Input: part model. Units: mm. Frame: model coordinates. Face numbers are marked on the shaded views. A direction names the side the tool comes from. Give positions to 0.01 mm unless a question says otherwise; leave off trailing zeros. Loops run counter-clockwise (first coordinate to the right, second up) from the corner with the lowest first, then second, coordinate; pieces in that order, holes last. Notation, with made-up numbers: (16.25, -19) - (57.25, -19) arc R13 cw to (57.25, 2) - close; hole circle Ø4 at (-38, 59.25). An arc over 180 degrees is marked (long way). One line per item, written item: value.
from build123d import *

# Parameters (mm, degrees)
ESBO_O1_W                = 37
ESBO_O1_H                = 17
RESSALTO_EXTRUS_O1_DEPTH = 0.45
ESBO_O2_W                = 10
ESBO_O2_H                = 11
RESSALTO_EXTRUS_O2_DEPTH = 5.1
RESSALTO_EXTRUS_O3_DEPTH = 5.1
ESBO_O4_W                = 4
ESBO_O4_H                = 1.5
CORTE_EXTRUS_O1_DEPTH    = 0.1
CHANFRO1_SIZE            = 1


with BuildPart() as part:
    # Esboço1 → Ressalto-extrusão1 (new, symmetric)
    with BuildSketch(Plane(origin=(0, 0, 0), x_dir=(1, 0, 0), z_dir=(0, 1, 0))):
        Rectangle(ESBO_O1_W, ESBO_O1_H)
    extrude(amount=RESSALTO_EXTRUS_O1_DEPTH, both=True)

    # Esboço2 → Ressalto-extrusão2 (add)
    with BuildSketch(Plane(origin=(0, 0.45, 0), x_dir=(1, 0, 0), z_dir=(0, 1, 0))):
        with Locations((-6.5, -2)):
            Rectangle(ESBO_O2_W, ESBO_O2_H)
    extrude(amount=RESSALTO_EXTRUS_O2_DEPTH)

    # Esboço3 → Ressalto-extrusão3 (add)
    with BuildSketch(Plane(origin=(0, 0.45, 0), x_dir=(1, 0, 0), z_dir=(0, 1, 0))):
        Polygon((0.5, 0.910833496), (0.5, 6.089166504), (1.910833496, 7.5), (8.967936907, 7.5), (9.5, 6.967936907), (9.5, 0.62041406), (8.37958594, -0.5), (1.910833496, -0.5), align=None)
    extrude(amount=RESSALTO_EXTRUS_O3_DEPTH)

    # Esboço4 → Corte-extrusão1 (cut)
    with BuildSketch(Plane(origin=(0, 0.45, 0), x_dir=(1, 0, 0), z_dir=(0, 1, 0))):
        with Locations((-15, 4.75)):
            Rectangle(ESBO_O4_W, ESBO_O4_H)
        with Locations((-15, -4.75)):
            Rectangle(ESBO_O4_W, ESBO_O4_H)
        with Locations((15, -4.75)):
            Rectangle(ESBO_O4_W, ESBO_O4_H)
        with Locations((15, 4.75)):
            Rectangle(ESBO_O4_W, ESBO_O4_H)
    extrude(amount=-CORTE_EXTRUS_O1_DEPTH, mode=Mode.SUBTRACT)

    # Chanfro1
    chanfro1_edges = [part.edges().sort_by_distance(p)[0] for p in [
        (-18.5, 0, -8.5),
        (18.5, 0, -8.5),
        (18.5, 0, 8.5),
        (-18.5, 0, 8.5),
    ]]
    chamfer(chanfro1_edges, length=CHANFRO1_SIZE)


solid = part.part
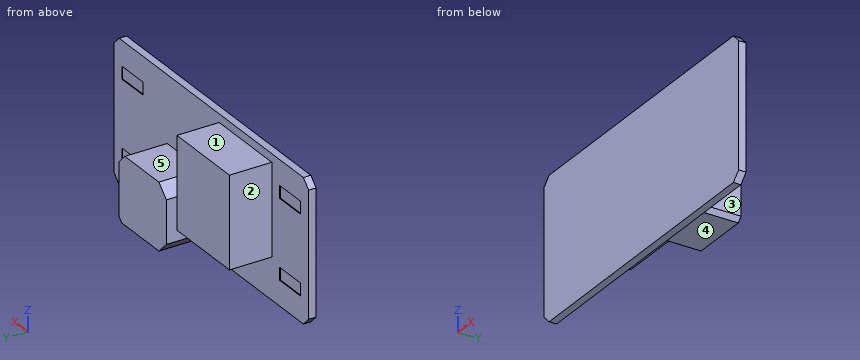
Item 1: Access query for the marked faces 1, 2, 3, 4 and 5. Directions: +Z, -Z, +X, -X, +Y, -Y. A direction counts if a zero-diameter tool reaches every point of the face in a straight line with its end or side. Return the directions, or none.
Verdict:
face 1: +Z, +X, -X, +Y
face 2: +Z, -Z, -X, +Y
face 3: +Z, -Z, +X, +Y
face 4: -Z, +X, -X, +Y
face 5: +Z, +X, +Y
Item 2: Section D-D, the plane z = 3.5. Output: boundary loops of the cut face in (x, y), and give its area (3 significant figures).
Verdict:
outline: (-18.5, -0.45) - (18.5, -0.45) - (18.5, 0.45) - (-1.5, 0.45) - (-1.5, 5.55) - (-11.5, 5.55) - (-11.5, 0.45) - (-18.5, 0.45) - close
area: 84.3 mm^2
Item 3: Section A-A, the plane y = 3.1. Output: boundary loops of the cut face in (x, z), and give its area (3 significant figures).
Verdict:
outline: (-11.5, -3.5) - (-1.5, -3.5) - (-1.5, 7.5) - (-11.5, 7.5) - close; (0.5, -6.09) - (1.91, -7.5) - (8.97, -7.5) - (9.5, -6.97) - (9.5, -0.62) - (8.38, 0.5) - (1.91, 0.5) - (0.5, -0.91) - close
area: 179 mm^2
Item 4: Section C-C, the plane z = -4.5. Output: boundary loops of the cut face in (x, y).
Verdict:
outline: (-18.5, -0.45) - (18.5, -0.45) - (18.5, 0.45) - (17, 0.45) - (17, 0.35) - (13, 0.35) - (13, 0.45) - (9.5, 0.45) - (9.5, 5.55) - (0.5, 5.55) - (0.5, 0.45) - (-13, 0.45) - (-13, 0.35) - (-17, 0.35) - (-17, 0.45) - (-18.5, 0.45) - close
Item 5: Section B-B, the plane x = 4. Output: boundary loops of the cut face in (y, z).
Verdict:
outline: (-0.45, -8.5) - (0.45, -8.5) - (0.45, -7.5) - (5.55, -7.5) - (5.55, 0.5) - (0.45, 0.5) - (0.45, 8.5) - (-0.45, 8.5) - close
Item 6: Pin query (flat end, axial travel): P1, Ø8, axis at x = -12, z = 1.5, coming from the +Y side; P2, Ø2.5, axis at x = -8.5, y = 4, coming from the +Z side; P3, Ø1.6, axis at x = 16, z = 4.5, coming from the +Y side; P4, Ø0.8, axis at x = -15.5, z = 5, coming from the +Y side. Return the tip coordinate at first contact, or that it passes through.
Verdict:
P1: stops at y = 5.55
P2: stops at z = 7.5
P3: stops at y = 0.45
P4: stops at y = 0.35
Item 7: Material intervals for L1, parallel to X at y = 2.1, z = -3; L2, parallel to Y at x = -16, z = 7.75; L3, parallel to X at y = 3.35, z = 0, sorted ascending.
Verdict:
L1: x = -11.5 to -1.5, 0.5 to 9.5
L2: y = -0.45 to 0.45
L3: x = -11.5 to -1.5, 1.41 to 8.88
